```python
from build123d import *

# Parameters (mm, degrees)
F0_R     = 15
F0_R_2   = 1
F1_DEPTH = 2
F3_DEPTH = 28
F5_DEPTH = 10
F7_DEPTH = 0.9
F9_DEPTH = 0.9
F10_R    = 1


with BuildPart() as f1:
    # F0 (on Top) → F1 (new body)
    with BuildSketch(Plane.XY):
        Circle(F0_R)
        with BuildLine():
            Line((0, -7), (0, -9))
            ThreePointArc((0, -9), (-1.17473573, -8.9230037524), (-2.3293714059, -8.6933324366))
            Line((-2.3293714059, -8.6933324366), (-1.8117333157, -6.761480784))
            ThreePointArc((-1.8117333157, -6.761480784), (-0.9136833455, -6.9401140296), (0, -7))
        make_face(mode=Mode.SUBTRACT)
        with BuildLine():
            Line((-3.5, -6.0621778265), (-4.5, -7.7942286341))
            ThreePointArc((-4.5, -7.7942286341), (-5.4788528611, -7.1401800626), (-6.3639610307, -6.3639610307))
            Line((-6.3639610307, -6.3639610307), (-4.9497474683, -4.9497474683))
            ThreePointArc((-4.9497474683, -4.9497474683), (-4.2613300031, -5.553473382), (-3.5, -6.0621778265))
        make_face(mode=Mode.SUBTRACT)
        with BuildLine():
            Line((-6.0621778265, -3.5), (-7.7942286341, -4.5))
            ThreePointArc((-7.7942286341, -4.5), (-8.3149157926, -3.4441508913), (-8.6933324366, -2.3293714059))
            Line((-8.6933324366, -2.3293714059), (-6.761480784, -1.8117333157))
            ThreePointArc((-6.761480784, -1.8117333157), (-6.4671567276, -2.6787840266), (-6.0621778265, -3.5))
        make_face(mode=Mode.SUBTRACT)
        with BuildLine():
            Line((-4.3301270189, -2.5), (-2.5980762114, -1.5))
            ThreePointArc((-2.5980762114, -1.5), (-2.1213203436, -2.1213203436), (-1.5, -2.5980762114))
            Line((-1.5, -2.5980762114), (-2.5, -4.3301270189))
            ThreePointArc((-2.5, -4.3301270189), (-3.5355339059, -3.5355339059), (-4.3301270189, -2.5))
        make_face(mode=Mode.SUBTRACT)
        with BuildLine():
            Line((3.5, -6.0621778265), (4.5, -7.7942286341))
            ThreePointArc((4.5, -7.7942286341), (3.4441508913, -8.3149157926), (2.3293714059, -8.6933324366))
            Line((2.3293714059, -8.6933324366), (1.8117333157, -6.761480784))
            ThreePointArc((1.8117333157, -6.761480784), (2.6787840266, -6.4671567276), (3.5, -6.0621778265))
        make_face(mode=Mode.SUBTRACT)
        with BuildLine():
            Line((0, -5), (0, -3))
            ThreePointArc((0, -3), (0.7764571353, -2.8977774789), (1.5, -2.5980762114))
            Line((1.5, -2.5980762114), (2.5, -4.3301270189))
            ThreePointArc((2.5, -4.3301270189), (1.2940952255, -4.8296291314), (0, -5))
        make_face(mode=Mode.SUBTRACT)
        with BuildLine():
            Line((6.0621778265, -3.5), (7.7942286341, -4.5))
            ThreePointArc((7.7942286341, -4.5), (7.1401800626, -5.4788528611), (6.3639610307, -6.3639610307))
            Line((6.3639610307, -6.3639610307), (4.9497474683, -4.9497474683))
            ThreePointArc((4.9497474683, -4.9497474683), (5.553473382, -4.2613300031), (6.0621778265, -3.5))
        make_face(mode=Mode.SUBTRACT)
        with BuildLine():
            Line((4.3301270189, -2.5), (2.5980762114, -1.5))
            ThreePointArc((2.5980762114, -1.5), (2.8977774789, -0.7764571353), (3, 0))
            Line((3, 0), (5, 0))
            ThreePointArc((5, 0), (4.8296291314, -1.2940952255), (4.3301270189, -2.5))
        make_face(mode=Mode.SUBTRACT)
        with BuildLine():
            Line((7, 0), (9, 0))
            ThreePointArc((9, 0), (8.9230037524, -1.17473573), (8.6933324366, -2.3293714059))
            Line((8.6933324366, -2.3293714059), (6.761480784, -1.8117333157))
            ThreePointArc((6.761480784, -1.8117333157), (6.9401140296, -0.9136833455), (7, 0))
        make_face(mode=Mode.SUBTRACT)
        with BuildLine():
            ThreePointArc((-6.761480784, 1.8117333157), (-6.9401140296, 0.9136833455), (-7, 0))
            Line((-7, 0), (-9, 0))
            ThreePointArc((-9, 0), (-8.9230037524, 1.17473573), (-8.6933324366, 2.3293714059))
            Line((-8.6933324366, 2.3293714059), (-6.761480784, 1.8117333157))
        make_face(mode=Mode.SUBTRACT)
        with BuildLine():
            ThreePointArc((-2.5980762114, 1.5), (-2.8977774789, 0.7764571353), (-3, 0))
            Line((-3, 0), (-5, 0))
            ThreePointArc((-5, 0), (-4.8296291314, 1.2940952255), (-4.3301270189, 2.5))
            Line((-4.3301270189, 2.5), (-2.5980762114, 1.5))
        make_face(mode=Mode.SUBTRACT)
        with BuildLine():
            Line((-6.0621778265, 3.5), (-7.7942286341, 4.5))
            ThreePointArc((-7.7942286341, 4.5), (-7.1401800626, 5.4788528611), (-6.3639610307, 6.3639610307))
            Line((-6.3639610307, 6.3639610307), (-4.9497474683, 4.9497474683))
            ThreePointArc((-4.9497474683, 4.9497474683), (-5.553473382, 4.2613300031), (-6.0621778265, 3.5))
        make_face(mode=Mode.SUBTRACT)
        with BuildLine():
            ThreePointArc((0, 3), (-0.7764571353, 2.8977774789), (-1.5, 2.5980762114))
            Line((-1.5, 2.5980762114), (-2.5, 4.3301270189))
            ThreePointArc((-2.5, 4.3301270189), (-1.2940952255, 4.8296291314), (0, 5))
            Line((0, 5), (0, 3))
        make_face(mode=Mode.SUBTRACT)
        with BuildLine():
            Line((-3.5, 6.0621778265), (-4.5, 7.7942286341))
            ThreePointArc((-4.5, 7.7942286341), (-3.4441508913, 8.3149157926), (-2.3293714059, 8.6933324366))
            Line((-2.3293714059, 8.6933324366), (-1.8117333157, 6.761480784))
            ThreePointArc((-1.8117333157, 6.761480784), (-2.6787840266, 6.4671567276), (-3.5, 6.0621778265))
        make_face(mode=Mode.SUBTRACT)
        Circle(F0_R_2, mode=Mode.SUBTRACT)
        with BuildLine():
            Line((4.3301270189, 2.5), (2.5980762114, 1.5))
            ThreePointArc((2.5980762114, 1.5), (2.1213203436, 2.1213203436), (1.5, 2.5980762114))
            Line((1.5, 2.5980762114), (2.5, 4.3301270189))
            ThreePointArc((2.5, 4.3301270189), (3.5355339059, 3.5355339059), (4.3301270189, 2.5))
        make_face(mode=Mode.SUBTRACT)
        with BuildLine():
            Line((6.0621778265, 3.5), (7.7942286341, 4.5))
            ThreePointArc((7.7942286341, 4.5), (8.3149157926, 3.4441508913), (8.6933324366, 2.3293714059))
            Line((8.6933324366, 2.3293714059), (6.761480784, 1.8117333157))
            ThreePointArc((6.761480784, 1.8117333157), (6.4671567276, 2.6787840266), (6.0621778265, 3.5))
        make_face(mode=Mode.SUBTRACT)
        with BuildLine():
            Line((3.5, 6.0621778265), (4.5, 7.7942286341))
            ThreePointArc((4.5, 7.7942286341), (5.4788528611, 7.1401800626), (6.3639610307, 6.3639610307))
            Line((6.3639610307, 6.3639610307), (4.9497474683, 4.9497474683))
            ThreePointArc((4.9497474683, 4.9497474683), (4.2613300031, 5.553473382), (3.5, 6.0621778265))
        make_face(mode=Mode.SUBTRACT)
        with BuildLine():
            Line((0, 7), (0, 9))
            ThreePointArc((0, 9), (1.17473573, 8.9230037524), (2.3293714059, 8.6933324366))
            Line((2.3293714059, 8.6933324366), (1.8117333157, 6.761480784))
            ThreePointArc((1.8117333157, 6.761480784), (0.9136833455, 6.9401140296), (0, 7))
        make_face(mode=Mode.SUBTRACT)
    extrude(amount=F1_DEPTH)

    # F2 (on face) → F3 (join)
    with BuildSketch(Plane.XY.offset(2)):
        with BuildLine():
            Line((6.6963757191, 8.7268867432), (5.4788528611, 7.1401800626))
            Line((5.4788528342, 7.1401800833), (9.4456195625, 4.0963729176))
            Line((9.4456195625, 4.0963729176), (9.9313862061, 4.7294363327))
            ThreePointArc((9.9313862061, 4.7294363327), (8.5507613173, 6.9198613349), (6.6963757191, 8.7268867432))
        make_face()
        with BuildLine():
            Line((1.9978528032, 10.8170506228), (1.5120861596, 10.1839872077))
            Line((1.5120861596, 10.1839872077), (5.4788528342, 7.1401800833))
            Line((5.4788528611, 7.1401800626), (6.6963757191, 8.7268867432))
            ThreePointArc((6.6963757191, 8.7268867432), (4.4709728986, 10.0503930938), (1.9978528032, 10.8170506228))
        make_face()
        with BuildLine():
            Line((-9.4456195625, -4.0963729176), (-9.9313862061, -4.7294363327))
            ThreePointArc((-9.9313862061, -4.7294363327), (-8.5507612755, -6.9198613865), (-6.6963756136, -8.7268868241))
            ThreePointArc((-6.6963756136, -8.7268868241), (-4.4709728379, -10.0503931208), (-1.9978528032, -10.8170506228))
            Line((-1.9978528032, -10.8170506228), (-1.5120861596, -10.1839872077))
            Line((-1.5120861596, -10.1839872077), (-5.47885283, -7.1401800865))
            Line((-5.47885283, -7.1401800865), (-9.4456195625, -4.0963729176))
        make_face()
    extrude(amount=F3_DEPTH)

    # F4 (on face) → F5 (join)
    with BuildSketch(Plane(origin=(3.9667667015, -3.043807145, 0), x_dir=(0.608761429, 0.7933533403, 0), z_dir=(0.7933533403, -0.608761429, 0))):
        Polygon((-4.5, 27.5), (-9, 30), (-9, 2), (-7.5, 11.6874175146), (-7.5, 27.5), align=None)
        Polygon((4.5, 27.5), (7.5, 27.5), (7.5, 11.6874175146), (9, 2), (9, 30), align=None)
    extrude(amount=-F5_DEPTH)

    # F6 (on face) → F7 (join)
    with BuildSketch(Plane(origin=(3.9667667015, -3.043807145, 0), x_dir=(0.608761429, 0.7933533403, 0), z_dir=(0.7933533403, -0.608761429, 0))):
        Polygon((-9, 2), (-4.5, 27.5), (-7.5, 27.5), (-7.5, 22.8047555536), align=None)
        Polygon((7.5, 22.8047555536), (7.5, 27.5), (4.5, 27.5), (9, 2), align=None)
    extrude(amount=-F7_DEPTH)

    # F8 (on face) → F9 (join)
    with BuildSketch(Plane(origin=(-3.9667667015, 3.043807145, 0), x_dir=(-0.608761429, -0.7933533403, 0), z_dir=(-0.7933533403, 0.608761429, 0))):
        Polygon((-9, 2), (-4.5, 27.5), (-7.5, 27.5), (-7.5, 11.6874175146), align=None)
        Polygon((7.5, 27.5), (4.5, 27.5), (9, 2), (7.5, 11.6874175146), align=None)
    extrude(amount=-F9_DEPTH)

    # F10
    f10_edges = [f1.edges().sort_by_distance(p)[0] for p in [
        (-15, 0, 0),
    ]]
    fillet(f10_edges, radius=F10_R)


solid = f1.part
```
Model file for the job. Use its own axes, mm. A direction names the side the tool comes from. Round coordinates to 2 decimals unless told otherwise and drop trailing zeros. Order: outer loops, then holes, each group sorted by start corner. A loop starts at its lowest first (then second) coordinate and runs counter-clockwise, first axis right, second up. Notation, with made-up numbers: (56, 15) -> (102, 15) arc R28 ccw to (102, 52) -> close; hole circle Ø2 at (7.5, -17.75). An arc over 180 degrees is marked (long way). Use one line per item in the form item = value.
Item 1: Cut at C-C, the plane z = 28.25. Write the cut outline in (x, y), and give its area (3 significant figures).
Returned:
outline = (-9.93, -4.73) arc R11 ccw to (-2, -10.82) -> (0.41, -7.68) -> (-7.53, -1.6) -> close; (-0.41, 7.68) -> (7.53, 1.6) -> (9.93, 4.73) arc R11 ccw to (2, 10.82) -> close
area = 95.2 mm^2
Item 2: Drill centre lines: line 1 (Y direction, x = -7.25, z = 1.75); line 2 (Z direction, x = -7.5, y = 4); line 3 (Y direction, x = 5, z = 2.5). Where is each one in solid material? Low to high.
Returned:
line_1 = -13.13 to -4.19, -1.94 to 0, 1.94 to 4.19, 5.33 to 13.13
line_2 = 0 to 2
line_3 = 7.41 to 9.8
Item 3: Pull direction X, two halves, no side cores. Call faces 1 (the face through (7.254, 2.719, 22.365)), 2 (the face through (0.77, -2.9, 0.99)), 3 (the face through (-7.254, -2.719, 22.365)): released by +X, released by -X, zero draft, split by the parting line, or undercut.
Returned:
face_1 = released by -X
face_2 = undercut
face_3 = released by +X
Item 4: Cut at A-A, the plane z = 24.75. Write the cut outline in (x, y).
Returned:
outline = (-9.93, -4.73) arc R11 ccw to (-2, -10.82) -> (0.93, -7) -> (0.22, -6.45) -> (-1.31, -8.45) -> (-7.82, -3.45) -> (-6.29, -1.46) -> (-7, -0.91) -> close; (-0.93, 7) -> (-0.22, 6.45) -> (1.31, 8.45) -> (7.82, 3.45) -> (6.29, 1.46) -> (7, 0.91) -> (9.93, 4.73) arc R11 ccw to (2, 10.82) -> close
Item 5: Tool access for faces 4 (the face through (-4.272, -5.546, 0.986)), 5 (the face through (-6.916, 3.993, 0.986)), 6 (the face through (-0.2, -2.9, 0)): list every direction of +Z, -Z, +X, -X, +Y, -Y with a clear straight run to the whole face (end or side of a thin tool).
Returned:
face_4 = -Z
face_5 = +Z, -Z
face_6 = -Z, +X, -X, +Y, -Y
Item 6: Flat gauge pins, fed straight in: pin 1 Ø1 at (x, z) = (-8.5, 0.5) entering from +Y; pin 2 Ø4 at (x, z) = (-5, 26) entering from +Y (3 decimals); pin 3 Ø2 at (y, z) = (-4, 1) entering from +X; pin 4 Ø1.6 at (x, y) = (0, 0) entering from +Z. Where does each tip first touch, or does it go through?
Returned:
pin_1 = 12.61
pin_2 = -0.605
pin_3 = 14.7
pin_4 = through
Item 7: Cut at B-B, the plane z = 9. Write the cut outline in (x, y).
Returned:
outline = (-9.93, -4.73) arc R11 ccw to (-2, -10.82) -> (-0.76, -9.2) -> (-1.47, -8.66) -> (-1.57, -8.78) -> (-8.07, -3.78) -> (-7.98, -3.66) -> (-8.69, -3.12) -> close; (0.76, 9.2) -> (1.47, 8.66) -> (1.57, 8.78) -> (8.07, 3.78) -> (7.98, 3.66) -> (8.69, 3.12) -> (9.93, 4.73) arc R11 ccw to (2, 10.82) -> close
